from build123d import *

# Parameters (mm, degrees)
BOSS_EXTRUDE1_DEPTH = 3.175
CHAMFER1_SIZE       = 2


with BuildPart() as part:
    # Sketch1 → Boss-Extrude1 (new body)
    with BuildSketch(Plane.XY):
        Polygon((-29.813098334, 12.635256228), (-24.517121596, 31.921329711), (-28.133260375, 32.914325349), (-33.429237113, 13.628251866), align=None)
        Polygon((0, 56.785184499), (0, -31.944815501), (-34.098545596, -2.970826443), (-19.692486788, 49.490942654), align=None)
        Polygon((0, 56.785184499), (19.692486788, 49.490942654), (34.098545596, -2.970826443), (0, -31.944815501), align=None)
        Polygon((28.133260375, 32.914325349), (24.517121596, 31.921329711), (29.813098334, 12.635256228), (33.429237113, 13.628251866), align=None)
        Polygon((-11.046183779, -25.183235467), (-9.751140598, -23.659141257), (-24.992082694, -10.708709448), (-26.287125875, -12.232803658), align=None)
        Polygon((26.287125875, -12.232803658), (11.046183779, -25.183235467), (9.751140598, -23.659141257), (24.992082694, -10.708709448), align=None)
    extrude(amount=BOSS_EXTRUDE1_DEPTH)

    # Chamfer1
    chamfer1_edges = [part.edges().sort_by_distance(p)[0] for p in [
        (18.666654827, -18.708019562, 0),
        (-18.666654827, -18.708019562, 0),
        (-30.781248744, 23.271288608, 0),
        (30.781248744, 23.271288608, 0),
    ]]
    chamfer(chamfer1_edges, length=CHAMFER1_SIZE)


solid = part.part
Model file for the job. Use its own axes, mm. A direction names the side the tool comes from. Give positions to 0.01 mm unless a question says otherwise; leave off trailing zeros. Loops run counter-clockwise (first coordinate to the right, second up) from the corner with the lowest first, then second, coordinate; pieces in that order, holes last.
Item 1: Slice it at B-B (y = 30). Write the cut outline in (x, z) (1 decimal).
Check values:
outline: (-28.9, 2) - (-26.9, 0) - (26.9, 0) - (28.9, 2) - (28.9, 3.2) - (-28.9, 3.2) - close
Item 2: Slice it at D-D (y = 21). Write the cut outline in (x, z) (3 decimals).
Check values:
outline: (-31.405, 2) - (-29.331, 0) - (29.331, 0) - (31.405, 2) - (31.405, 3.175) - (-31.405, 3.175) - close
Item 3: Drop flat-ended pins along their axis: P1, Ø1, axis at x = -20, z = 0.5, coming from the +Y side; P2, Ø1, axis at x = -9.5, z = 0.5, coming from the +Y side; P3, Ø1.5, axis at y = -8, z = 1.5, coming from the +X side. Give the stop position or say it passes through.
Check values:
P1: stops at y = 49.56
P2: stops at y = 53.45
P3: stops at x = 29.06
Item 4: Drill centre lines: line 1 along X through (y, z) = (-25, 2.6); line 2 along X through (y, z) = (-16, 0.6); line 3 along X through (y, z) = (-13, 0.9). Where is each one in solid material? Low to high.
Check values:
line 1: x = -11.26 to -10.89, -8.17 to 8.17, 10.89 to 11.26
line 2: x = -19.69 to 19.69
line 3: x = -23.69 to 23.69
Item 5: Which spindle directions (+Z, -Z, +X, -X, +Y, -Y) get a long thin tool onto all of the face, cutting with end or side? Do faces 1 (the face through (-31.986, 4.723, 1.565)), 2 (the face through (25.9, 32.3, 1.9)), 3 (the face through (-4.81, -27.86, 1.57)), 4 (the face through (31.194, 13.014, 1.918)). Say none if no direction does.
Check values:
face 1: +Z, -Z, -X
face 2: +Z, -Z, +Y
face 3: +Z, -Z, -Y
face 4: +Z, -Z, +X
Item 6: Mould opens along X. For faces 5 (the face through (0, 13, 3.175)), 6 (the face through (31.926, 4.941, 1.565)), 7 (the face through (-25.9, 32.3, 1.9)), 8 (the face through (-31.245, 13.028, 1.918)) say: +X half, -X half, draft (parallel to the pull), parting line (faces both ways), or undercut.
Check values:
face 5: draft
face 6: +X half
face 7: undercut
face 8: -X half
Item 7: Slice it at C-C (x = 3). Write the cut outline in (y, z) (3 decimals), plus the area to 3 significant figures.
Check values:
outline: (-29.396, 0) - (55.674, 0) - (55.674, 3.175) - (-29.396, 3.175) - close
area: 270 mm2
Item 8: Slice it at A-A (z = 2.6). Write the cut outline in (x, y).
Check values:
outline: (-34.1, -2.97) - (-24.99, -10.71) - (-26.29, -12.23) - (-11.05, -25.18) - (-9.75, -23.66) - (0, -31.94) - (9.75, -23.66) - (11.05, -25.18) - (26.29, -12.23) - (24.99, -10.71) - (34.1, -2.97) - (29.81, 12.64) - (33.43, 13.63) - (28.13, 32.91) - (24.52, 31.92) - (19.69, 49.49) - (0, 56.79) - (-19.69, 49.49) - (-24.52, 31.92) - (-28.13, 32.91) - (-33.43, 13.63) - (-29.81, 12.64) - close
